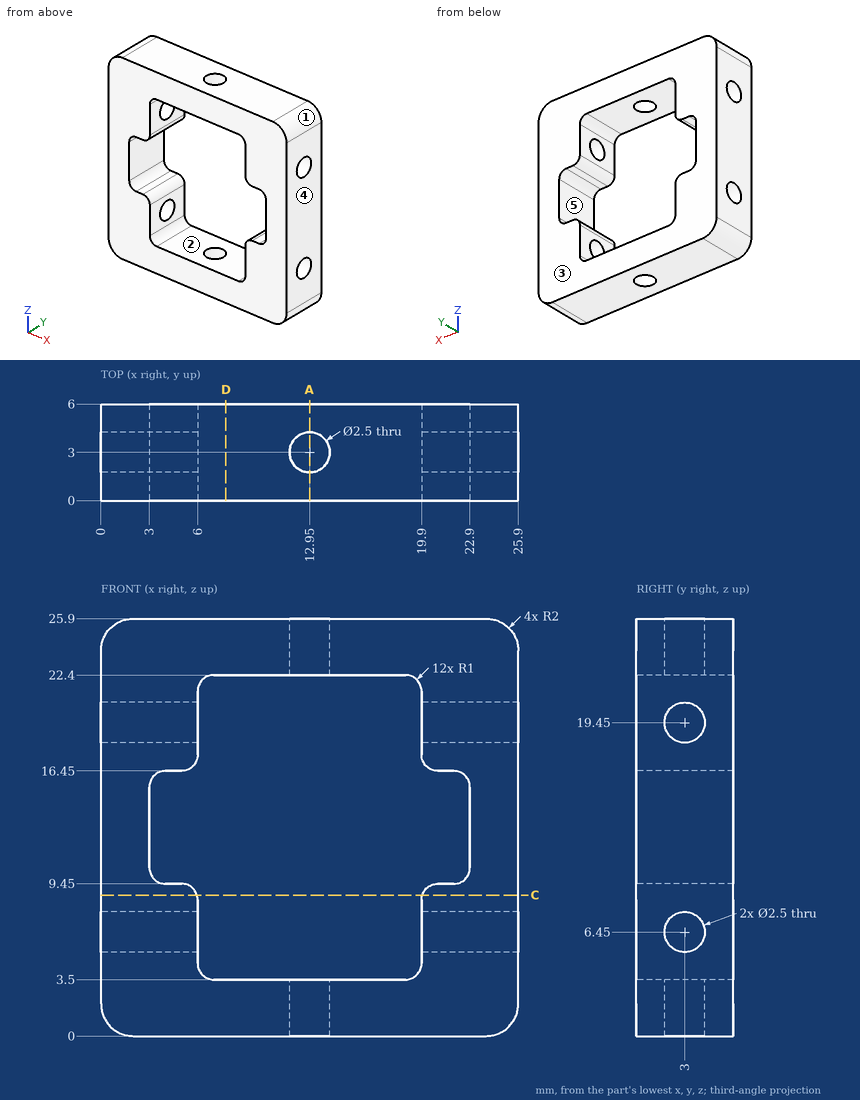
Could you check a few things on this drawing? It's one solid part, dimensions in mm from its lowest x, y, z. A direction names the side the tool comes from. Coordinates: 2 decimals unless noted, no trailing zeros. Order: outer loops, then holes, each group sorted by start corner. A loop starts at its lowest first (then second) coordinate and runs counter-clockwise, first axis right, second up.
1. I need wall thicknesses on line 1 (Z direction, x = 22, y = 0.3); line 2 (Z direction, x = 14, y = 1.1); line 3 (X direction, y = 4.75, z = 15). Which ranges of each line are inside material? Lowest first, please.
2. For the marked faces 1 and 2, which set-ups out of +Z, -Z, +X, -X, +Y, -Y let a thin tool reach every point of the face, with its end or its side?
3. If we section it at C-C (z = 8.75): Please give me the cut outline in (x, y), then the cut area to 3 significant figures.
4. If we section it at A-A (x = 12.95): Please give me the cut outline in (y, z), then the cut area to 3 significant figures.
5. If we section it at D-D (x = 7.75): Please give me the cut outline in (y, z).
6. I'm going to push a flat-ended pin straight in: pin 1 (2 mm diameter, centred on x = 12.95, y = 3, fed in from -Z). Where does the tip first touch, or does it pass through?
7. Thinking about a two-plate mould opening in X: for the marked faces 3, 4 and 5, which applies, +X half, -X half, draft (parallel to the pull), parting line (faces both ways), or undercut?
Entries:
1. line 1: z = 0 to 9.46, 16.44 to 25.9
1. line 2: z = 0 to 3.5, 22.4 to 25.9
1. line 3: x = 0 to 3, 22.9 to 25.9
2. face 1: +Z, +X, +Y, -Y
2. face 2: +Y, -Y
3. outline: (0, 0) - (5.95, 0) - (5.95, 6) - (0, 6) - close; (19.95, 0) - (25.9, 0) - (25.9, 6) - (19.95, 6) - close
3. area: 71.4 mm2
4. outline: (0, 0) - (1.75, 0) - (1.75, 3.5) - (0, 3.5) - close; (0, 22.4) - (1.75, 22.4) - (1.75, 25.9) - (0, 25.9) - close; (4.25, 0) - (6, 0) - (6, 3.5) - (4.25, 3.5) - close; (4.25, 22.4) - (6, 22.4) - (6, 25.9) - (4.25, 25.9) - close
4. area: 24.5 mm2
5. outline: (0, 0) - (6, 0) - (6, 3.5) - (0, 3.5) - close; (0, 22.4) - (6, 22.4) - (6, 25.9) - (0, 25.9) - close
6. pin 1: passes through
7. face 3: draft
7. face 4: +X half
7. face 5: undercut
